The listing builds one solid part. Answer for the finished solid, in the listing's coordinates (mm). A direction names the side the tool comes from. Round coordinates to 2 decimals unless told otherwise and drop trailing zeros. Order: outer loops, then holes, each group sorted by start corner. A loop starts at its lowest first (then second) coordinate and runs counter-clockwise, first axis right, second up. Notation, with made-up numbers: (28, 81) - (80, 81) arc R20 ccw to (80, 113) - close; hole circle Ø9 at (7, 71). An arc over 180 degrees is marked (long way). One line per item, written item: value. Start each with the question number.
1. Straight lines are drawn through the part: line 1 (Z direction, x = 0, y = -1.15); line 2 (Z direction, x = 0, y = -5.25); line 3 (Y direction, x = 17, z = 1). For each, find the intervals that lie inside material, in ascending order.
2. A tool of negligible diameter and unlimited length cuts with its end or side. For faces 1 (the cylindrical face through (-20.43, -10.48, -0.65)), 2 (the flat face through (30, -5, 0)), 3 (the cylindrical face through (-28.57, -5.55, 11)), 4 (the cylindrical face through (-6, -1, 0)), from which of +Z, -Z, +X, -X, +Y, -Y can it reach the whole face along a straight path? Write none if from no direction.
3. For a pull along Z with two mould halves and no side action, classify faces 5 (the flat face through (42.5, -1, -5)), 6 (the cylindrical face through (-14.93, -10.48, -5.15)), 7 (the cylindrical face through (39.49, -1.01, -32.15)) as released by +Z, released by -Z, zero draft, split by the parting line, or undercut.
4. Section A-A, the plane x = 0 is taken. Give the vertices of the cut face in (y, z).
5. Flat-ended cylindrical pins translate along their axes: P1, Ø12.5, axis at x = 0, z = 0, coming from the +Y side; P2, Ø5, axis at y = -10.5, z = 10, coming from the +X side; P3, Ø3.5, axis at x = 3.5, y = -5.5, coming from the -Z side; P4, Ø6, axis at x = -17, z = 10, coming from the -Y side. Find the tip coordinate at first contact, or state that the pin passes through.
6. Section D-D, the plane y = -1 is taken. Give the vertices of the cut face in (x, z), then the cut area to 3 significant figures.
7. Section C-C, the plane y = -10 is taken. Give the vertices of the cut face in (x, z).
from build123d import *

# Parameters (mm, degrees)
F0_W     = 85
F0_H     = 60
F0_R     = 6
F1_DEPTH = 2
F2_W     = 60
F2_H     = 25
F2_R     = 5.5
F3_DEPTH = 7
F4_R     = 5
F5_R     = 10
F6_R     = 1.7
F7_DEPTH = 3


with BuildPart() as f1:
    # F0 (on Front) → F1 (new body)
    with BuildSketch(Plane.XZ):
        with Locations((0, -5)):
            Rectangle(F0_W, F0_H)
        Circle(F0_R, mode=Mode.SUBTRACT)
    extrude(amount=F1_DEPTH)

    # F2 (on face) → F3 (join)
    with BuildSketch(Plane.XZ.offset(2)):
        Rectangle(F2_W, F2_H)
        Circle(F2_R, mode=Mode.SUBTRACT)
    extrude(amount=F3_DEPTH)

    # F4
    f4_edges = [f1.edges().sort_by_distance(p)[0] for p in [
        (30, -5.5, 12.5),
        (30, -5.5, -12.5),
        (-30, -5.5, -12.5),
        (-30, -5.5, 12.5),
    ]]
    fillet(f4_edges, radius=F4_R)

    # F5
    f5_edges = [f1.edges().sort_by_distance(p)[0] for p in [
        (42.5, -1, 25),
        (42.5, -1, -35),
        (-42.5, -1, -35),
        (-42.5, -1, 25),
    ]]
    fillet(f5_edges, radius=F5_R)

    # F6 (on face) → F7 (join)
    with BuildSketch(Plane.XZ.offset(9)):
        with Locations((-11, 0)):
            Circle(F6_R)
        with Locations((-22, 0)):
            Circle(F6_R)
        with Locations((11, 0)):
            Circle(F6_R)
        with Locations((22, 0)):
            Circle(F6_R)
        with Locations((-16.5, -4.5)):
            Circle(F6_R)
        with Locations((16.5, -4.5)):
            Circle(F6_R)
        with Locations((16.5, 4.5)):
            Circle(F6_R)
        with Locations((-16.5, 4.5)):
            Circle(F6_R)
    extrude(amount=F7_DEPTH)


solid = f1.part
Answer list:
1. line 1: z = -35 to -6, 6 to 25
1. line 2: z = -12.5 to -5.5, 5.5 to 12.5
1. line 3: y = -9 to 0
2. face 1: -Y
2. face 2: +Z, -Z, +X, -Y
2. face 3: +Z, -X, -Y
2. face 4: +Y
3. face 5: zero draft
3. face 6: undercut
3. face 7: released by -Z
4. outline: (-9, -12.5) - (-2, -12.5) - (-2, -35) - (0, -35) - (0, -6) - (-2, -6) - (-2, -5.5) - (-9, -5.5) - close; (-9, 5.5) - (-2, 5.5) - (-2, 6) - (0, 6) - (0, 25) - (-2, 25) - (-2, 12.5) - (-9, 12.5) - close
5. P1: stops at y = 0
5. P2: stops at x = 29.97
5. P3: stops at z = -12.5
5. P4: stops at y = -9
6. outline: (-42.5, -25) arc R10 ccw to (-32.5, -35) - (32.5, -35) arc R10 ccw to (42.5, -25) - (42.5, 15) arc R10 ccw to (32.5, 25) - (-32.5, 25) arc R10 ccw to (-42.5, 15) - close; hole circle Ø12 at (0, 0)
6. area: 4,900 mm²
7. outline: circle Ø3.4 at (-22, 0); circle Ø3.4 at (-16.5, -4.5); circle Ø3.4 at (-16.5, 4.5); circle Ø3.4 at (-11, 0); circle Ø3.4 at (11, 0); circle Ø3.4 at (16.5, -4.5); circle Ø3.4 at (16.5, 4.5); circle Ø3.4 at (22, 0)
